Could you check a few things on this model? Use its own coordinates, in mm. Face numbers are marked on the shaded views. A direction names the side the tool comes from. Round coordinates to 2 decimals unless told otherwise and drop trailing zeros. Write each loop counter-clockwise with the first axis right and the second up, starting at its lowest first coordinate (ties: lowest second). Pieces come first, ordered by that corner, then holes. Notation, with made-up numbers: (-25.5, 31.5) -> (-20.5, 31.5) arc R26 ccw to (-20.5, 47.5) -> close; hole circle Ø6 at (72, 47). An arc over 180 degrees is marked (long way). One line per question, with ' | ' between items. Start each with the question number.
1. For pin 1 Ø1 at (x, y) = (-4.5, 5) entering from +Z; pin 2 Ø4 at (x, y) = (-6.5, 9) entering from +Z; pin 3 Ø1 at (y, z) = (13.5, 6) entering from -X, each with a flat end and sliding along its axis, tell me the tip position at first contact or that it passes through.
2. Thinking about a two-plate mould opening in Z: for the marked faces 1, 2 and 3, which applies, released by +Z, released by -Z, zero draft, split by the parting line, or undercut?
3. For the marked faces 4, 5 and 6, which set-ups out of +Z, -Z, +X, -X, +Y, -Y let a thin tool reach every point of the face, with its end or its side?
4. Imagine slicing it at C-C, the plane x = -5.75. List the corners of the cut face in (y, z) for me, and give its area (3 significant figures).
5. Imagine slicing it at B-B, the plane y = 8.25. List the corners of the cut face in (x, z) for me, and give its area (3 significant figures).
6. Imagine slicing it at A-A, the plane y = 1.5. List the corners of the cut face in (x, z) for me.
7. Imagine slicing it at D-D, the plane z = -8.75. List the corners of the cut face in (x, y) for me.
8. If I drill on line 1 along Y through (x, z) = (-2.5, -7.5); line 2 along Z through (x, y) = (0, 9.5); line 3 along Z through (x, y) = (6.25, 3.75), over which ranges is the centre line in solid material (lowest first)? Write a range as [from, to].
Autodesk Inventor part; units mm, degrees
ref_plane "YZ Plane" through (0, 0, 0) normal (1, 0, 0) x (0, 1, 0)
ref_plane "XZ Plane" through (0, 0, 0) normal (0, 1, 0) x (-1, 0, 0)
ref_plane "XY Plane" through (0, 0, 0) normal (0, 0, 1) x (1, 0, 0)
sketch "Sketch1" plane through (0, 0, 0) normal (0, 1, 0) x (-1, 0, 0)
  circle A0 centre (0, 0) radius 12 construction
  line L0 (8.75, -7) -> (5, -7)
  line L1 (8.75, 7) -> (5, 7)
  line L2 (-5, 7) -> (-8.75, 7)
  line L3 (-5.25, -6.7253) -> (-9, -6.7253)
  line L4 (8.75, -7) -> (8.75, -8.212)
  line L5 (8.75, 7) -> (8.75, 8.212)
  line L6 (-8.75, 7) -> (-8.75, 8.212)
  arc A1 (8.75, 8.212) -> (-8.75, 8.212) centre (0, 0) ccw
  arc A2 (5, 7) -> (-5, 7) centre (0, 3.6834) ccw
  line L7 (-9, -6.7253) -> (-9, -7.9373)
  arc A3 (-9, -7.9373) -> (8.75, -8.212) centre (0, 0) ccw
  arc A4 (-5.25, -6.7253) -> (5, -7) centre (-0.0415, -3.7468) ccw
  circle A5 centre (0, 0) radius 4.75
  circle A6 centre (0, 0) radius 3
  line L8 (5, 7) -> (5, -7)
  line L9 (-5, 7) -> (-5.25, -6.7253)
  dimension "d0" = 24
  dimension "d2" = 3.75
  dimension "d3" = 3.75
  dimension "d5" = 3.75
  dimension "d6" = 3.75
  dimension "d28" = 8.75
  dimension "d29" = 14
  dimension "d31" = 1.212
  dimension "d32" = 1.212
  dimension "d33" = 6
  dimension "d34" = 1.212
  dimension "d35" = 1.212
  dimension "d49" = 9.5
  dimension "d50" = 6
  dimension "d51" = 1.044
extrude "Extrusion3" add sketch "Sketch1" along normal blind 16 contours A4 L9 A2 L8
extrude "Extrusion5" add sketch "Sketch1" along normal blind 17 contours L4 A3 L7 L3 A4 L0 | A2 L2 L6 A1 L5 L1 | A5
sketch "Sketch2" plane through (5.25, 0, -6.7253) normal (0.9998342, 0, 0.0182116) x (0.0182116, 0, -0.9998342)
  line L0 (-13.7275, 0) -> (0, 0)
  line L1 (0, 0) -> (0, 16)
  line L2 (-13.7275, 16) -> (0, 16)
  line L3 (-13.7275, 0) -> (-13.7275, 16)
  circle A0 centre (-6.8638, 6) radius 3
  line L4 (2.9272, 16) -> (0, 16)
  line L5 (0.0881, 0) -> (-13.9096, 0)
  line L6 (-13.9096, 0) -> (-13.9096, 16)
  line L7 (0.0881, 16) -> (-13.9096, 16)
  line L8 (0.0881, 0) -> (0.0881, 16)
  point P0 (-6.8197, 0)
  dimension "d54" = 6
  dimension "d55" = 6
extrude "Extrusion6" cut sketch "Sketch2" against normal through all contours A0
fillet "Fillet1" radius 2 1 edges at (4.75, 16, 0)
properties part number "reverse gear cross head 1"
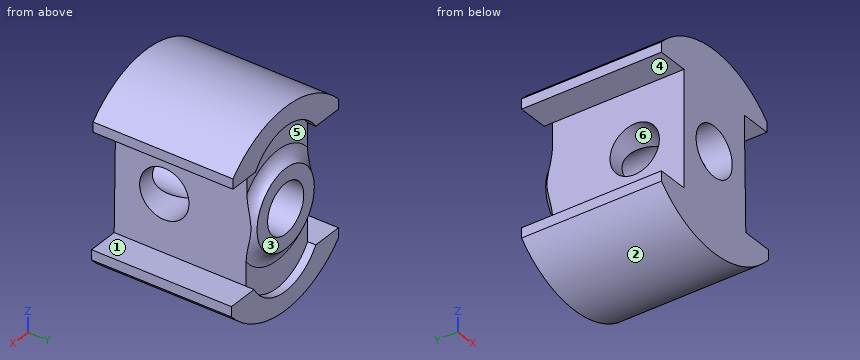
Geometry results:
1) pin 1: stops at z = 11.31 | pin 2: stops at z = 11.12 | pin 3: stops at x = -5
2) face 1: undercut | face 2: released by -Z | face 3: zero draft
3) face 4: -X, +Y, -Y | face 5: +Y | face 6: none
4) outline: (0, -10.53) -> (17, -10.53) -> (17, -7) -> (0, -7) -> close; (0, 7) -> (17, 7) -> (17, 10.53) -> (0, 10.53) -> close | area: 120 mm2
5) outline: (-8.75, -8.21) arc R12 ccw to (9, -7.94) -> (9, -6.73) -> (5.25, -6.73) -> (5.16, -1.85) -> (2.32, -1.9) arc R3 cw to (-2.25, -1.98) -> (-5, -2.03) -> (-5, -7) -> (-8.75, -7) -> close; (-8.75, 7) -> (-5, 7) -> (-5, 1.94) -> (-2.25, 1.99) arc R3 cw to (2.17, 2.07) -> (5.09, 2.12) -> (5, 7) -> (8.75, 7) -> (8.75, 8.21) arc R12 ccw to (-8.75, 8.21) -> close | area: 231 mm2
6) outline: (-8.75, -8.21) arc R12 ccw to (9, -7.94) -> (9, -6.73) -> (5.25, -6.73) -> (5, 7) -> (8.75, 7) -> (8.75, 8.21) arc R12 ccw to (-8.75, 8.21) -> (-8.75, 7) -> (-5, 7) -> (-5, -7) -> (-8.75, -7) -> close; hole circle Ø6 at (0, 0)
7) outline: (-8.21, 0) -> (8.21, 0) -> (8.21, 17) -> (3.35, 17) -> (3.35, 16) -> (-3.27, 16) -> (-3.27, 17) -> (-8.21, 17) -> close
8) line 1: y = [0, 16] | line 2: z = [-12, -3], [3, 12] | line 3: z = [-10.24, -6.73], [7, 10.24]
